from build123d import *

# Parameters (mm, degrees)
SKETCH1_W           = 20
SKETCH1_H           = 20
BOSS_EXTRUDE1_DEPTH = 5
FILLET1_R           = 3
CUT_EXTRUDE1_REACH  = 19.321
SKETCH2_R           = 5
SKETCH3_R           = 6.5
CUT_EXTRUDE2_DEPTH  = 5


with BuildPart() as part:
    # Sketch1 → Boss-Extrude1 (new, symmetric)
    with BuildSketch(Plane.XY):
        Rectangle(SKETCH1_W, SKETCH1_H)
    extrude(amount=BOSS_EXTRUDE1_DEPTH, both=True)

    # Fillet1
    fillet1_edges = [part.edges().sort_by_distance(p)[0] for p in [
        (10, -10, 0),
        (-10, -10, 0),
        (-10, 10, 0),
        (10, 10, 0),
    ]]
    fillet(fillet1_edges, radius=FILLET1_R)

    # Sketch2 → Cut-Extrude1 (cut, up to next)
    with BuildSketch(Plane.XY.offset(5), mode=Mode.PRIVATE) as cut_extrude1_sk1:
        Circle(SKETCH2_R)
    cut_extrude1_tool1 = extrude(cut_extrude1_sk1.sketch, amount=-CUT_EXTRUDE1_REACH, mode=Mode.PRIVATE) & part.part
    add(cut_extrude1_tool1.solids().sort_by_distance((0, 0, 5))[0], mode=Mode.SUBTRACT)

    # Sketch3 → Cut-Extrude2 (cut)
    with BuildSketch(Plane.XY.offset(5)):
        Circle(SKETCH3_R)
    extrude(amount=-CUT_EXTRUDE2_DEPTH, mode=Mode.SUBTRACT)


solid = part.part
Build history of the part. All positions in model axes, mm. A direction names the side the tool comes from. Give positions to 0.01 mm unless a question says otherwise; leave off trailing zeros. Order: outer loops, then holes, each group sorted by start corner. A loop starts at its lowest first (then second) coordinate and runs counter-clockwise, first axis right, second up. Notation, with made-up numbers: M -13,78.25 L -7,78.25 A5 ccw -7,82.25 Z; hole C 70.5,29.5 d3. An arc over 180 degrees is marked long. Put each result on its own line as item: value.
Item 1: Which spindle directions (+Z, -Z, +X, -X, +Y, -Y) get a long thin tool onto all of the face, cutting with end or side? Do faces 4 (the face through (0, 10, 0)), 5 (the face through (2, -5, 0)). Say none if no direction does.
Results are:
face 4: +Z, -Z, +X, -X, +Y
face 5: +Z
Item 2: Pull direction X, two halves, no side cores. Call faces 1 (the face through (-9.14, -9.1, 0.07)), 2 (the face through (-5.158, -3.955, 2.535)), 3 (the face through (9.14, 9.1, -0.07)): +X half, -X half, draft (parallel to the pull), parting line (faces both ways), or undercut.
Results are:
face 1: -X half
face 2: undercut
face 3: +X half
Item 3: Drop flat-ended pins along their axis: pin 1 Ø8 at (x, y) = (0, 0) entering from -Z; pin 2 Ø6.5 at (x, y) = (3, -0.5) entering from +Z. Give the stop position or say it passes through.
Results are:
pin 1: through
pin 2: z = 0
Item 4: Cut at B-B on y = 0. Write the cut outline in (x, z).
Results are:
outline: M -10,-5 L -5,-5 L -5,0 L -6.5,0 L -6.5,5 L -10,5 Z; M 5,-5 L 10,-5 L 10,5 L 6.5,5 L 6.5,0 L 5,0 Z
Item 5: Cut at A-A on z = 4. Write the cut outline in (x, y), then the cut area to 3 significant figures.
Results are:
outline: M -10,-7 A3 ccw -7,-10 L 7,-10 A3 ccw 10,-7 L 10,7 A3 ccw 7,10 L -7,10 A3 ccw -10,7 Z; hole C 0,0 d13
area: 260 mm2
Item 6: Cut at D-D on y = -6. Write the cut outline in (x, z).
Results are:
outline: M -10,-5 L 10,-5 L 10,5 L 2.5,5 L 2.5,0 L -2.5,0 L -2.5,5 L -10,5 Z
Item 7: Wall check: probe 1 along Y at (x, z) = (0, -3); probe 2 along Y at (x, z) = (-0.25, 0.5); probe 3 along Z at (x, y) = (5, -2). Give the ranges that are in metal, low to high.
Results are:
probe 1: -10 to -5, 5 to 10
probe 2: -10 to -6.5, 6.5 to 10
probe 3: -5 to 0
